Could you check a few things on this model? Use its own coordinates, in mm. A direction names the side the tool comes from. Round coordinates to 2 decimals unless told otherwise and drop trailing zeros. Loops run counter-clockwise (first coordinate to the right, second up) from the corner with the lowest first, then second, coordinate; pieces in that order, holes last. Notation, with made-up numbers: (34.25, 71.5) -> (62.25, 71.5) arc R21 cw to (62.25, 83.5) -> close; hole circle Ø3 at (69.5, -20.75). An arc over 180 degrees is marked (long way). One line per item, written item: value.
from build123d import *

# Parameters (mm, degrees)
F0_R     = 15.5
F1_DEPTH = 6
F2_R     = 13.2
F3_DEPTH = 4
F5_DEPTH = 25


with BuildPart() as f1:
    # F0 (on Top) → F1 (new body)
    with BuildSketch(Plane.XY):
        Circle(F0_R)
    extrude(amount=F1_DEPTH)

    # F2 (on face) → F3 (cut)
    with BuildSketch(Plane.XY.offset(6)):
        Circle(F2_R)
    extrude(amount=-F3_DEPTH, mode=Mode.SUBTRACT)

    # F4 (on face) → F5 (cut)
    with BuildSketch(Plane.XY.offset(6)):
        with BuildLine():
            Line((6.95, 21.574851), (-6.95, 21.574851))
            Line((-6.95, 21.574851), (-6.95, 10.710004))
            ThreePointArc((-6.95, 10.710004), (0, 12.767407), (6.95, 10.710004))
            Line((6.95, 10.710004), (6.95, 21.574851))
        make_face()
    extrude(amount=-F5_DEPTH, mode=Mode.SUBTRACT)


solid = f1.part
(1) If we section it at B-B, the plane y = 0: Please give me the cut outline in (x, z).
Recorded:
outline: (-15.5, 0) -> (15.5, 0) -> (15.5, 6) -> (13.2, 6) -> (13.2, 2) -> (-13.2, 2) -> (-13.2, 6) -> (-15.5, 6) -> close
(2) I'm going to push flat-ended pins straight in: pin 1 Ø3 at (x, y) = (-2.5, -1) entering from -Z; pin 2 Ø1.5 at (x, z) = (-3, 1.5) entering from +Y; pin 3 Ø2 at (x, z) = (5, 4) entering from -Y (3 decimals); pin 4 Ø2.5 at (y, z) = (13, 2.5) entering from +X. Where does each tip first touch, or does it pass through?
Recorded:
pin 1: z = 0
pin 2: y = 12.57
pin 3: y = -14.975
pin 4: x = 10.11
(3) For faces 4 (the face through (-0.58, -15.49, 2.96)), 5 (the face through (0, 0, 2)), which set-ups out of +Z, -Z, +X, -X, +Y, -Y let a thin tool reach every point of the face, with its end or its side?
Recorded:
face 4: +Z, -Z
face 5: +Z
(4) If we section it at A-A, the plane x = 0: Please give me the cut outline in (y, z).
Recorded:
outline: (-15.5, 0) -> (12.77, 0) -> (12.77, 2) -> (-13.2, 2) -> (-13.2, 6) -> (-15.5, 6) -> close
(5) If we section it at C-C, the plane z = 5.6: Please give me the cut outline in (x, y).
Recorded:
outline: (-6.95, 11.22) -> (-6.95, 13.85) arc R15.5 ccw (long way) to (6.95, 13.85) -> (6.95, 11.22) arc R13.2 cw (long way) to start
(6) Thinking about a two-plate mould opening in Z: for faces 1 (the face through (-0.48, -13.19, 4.03)), 2 (the face through (0, -1, 0)), 3 (the face through (-5, -13, 6)), which applies, released by +Z, released by -Z, zero draft, split by the parting line, or undercut?
Recorded:
face 1: zero draft
face 2: released by -Z
face 3: released by +Z
(7) If I drill on L1, parallel to X at y = 0, z = 3.15; L2, parallel to Y at x = 0, z = 4.95; L3, parallel to Z at x = 1, y = 2.25, over which ranges is the centre line in solid material (lowest first)?
Recorded:
L1: -15.5 to -13.2, 13.2 to 15.5
L2: -15.5 to -13.2
L3: 0 to 2
(8) If we section it at D-D, the plane y = 10: Please give me the cut outline in (x, z), then the cut area to 3 significant figures.
Recorded:
outline: (-11.84, 0) -> (11.84, 0) -> (11.84, 6) -> (8.62, 6) -> (8.62, 2) -> (-8.62, 2) -> (-8.62, 6) -> (-11.84, 6) -> close
area: 73.2 mm²
